from build123d import *

# Parameters (mm, degrees)
F0_W     = 38.1
F0_H     = 3.175
F1_DEPTH = 15.875
F2_W     = 38.1
F2_H     = 3.175
F3_DEPTH = 2.54
F5_DEPTH = 25.4
F6_R     = 3.2385
F7_DEPTH = 101.6


with BuildPart() as f1:
    # F0 (on Top) → F1 (new body)
    with BuildSketch(Plane.XY):
        with BuildLine():
            Line((-43.00682, 50.395912), (-46.18182, 50.395912))
            Line((-46.18182, 50.395912), (-46.18182, -35.329088))
            ThreePointArc((-46.18182, -35.329088), (-44.321948, -39.819216), (-39.83182, -41.679088))
            Line((-39.83182, -41.679088), (-39.83182, -38.504088))
            ThreePointArc((-39.83182, -38.504088), (-42.076884, -37.574152), (-43.00682, -35.329088))
            Line((-43.00682, -35.329088), (-43.00682, 50.395912))
        make_face()
        with Locations((-20.78182, -40.091588)):
            Rectangle(F0_W, F0_H)
        with BuildLine():
            Line((-1.73182, -38.504088), (-1.73182, -41.679088))
            ThreePointArc((-1.73182, -41.679088), (2.758308, -39.819216), (4.61818, -35.329088))
            Line((4.61818, -35.329088), (4.61818, 50.395912))
            Line((4.61818, 50.395912), (1.44318, 50.395912))
            Line((1.44318, 50.395912), (1.44318, -35.329088))
            ThreePointArc((1.44318, -35.329088), (0.513244, -37.574152), (-1.73182, -38.504088))
        make_face()
    extrude(amount=F1_DEPTH)

    # F2 (on face) → F3 (join)
    with BuildSketch(Plane.XY.offset(15.875)):
        with Locations((-20.78182, -40.091588)):
            Rectangle(F2_W, F2_H)
    extrude(amount=F3_DEPTH)

    # F4 (on face) → F5 (cut)
    with BuildSketch(Plane.XZ.offset(41.679088)):
        Polygon((-39.83182, 18.415), (-39.83182, 15.875), (-37.29182, 18.415), align=None)
        Polygon((-1.73182, 18.415), (-4.207504, 18.415), (-1.73182, 15.875), align=None)
    extrude(amount=-F5_DEPTH, mode=Mode.SUBTRACT)

    # F6 (on face) → F7 (cut)
    with BuildSketch(Plane(origin=(-46.18182, 0, 0), x_dir=(0, -1, 0), z_dir=(-1, 0, 0))):
        with Locations((-42.471112, 7.9502)):
            Circle(F6_R)
    extrude(amount=-F7_DEPTH, mode=Mode.SUBTRACT)


solid = f1.part
Read the model definition and answer for the solid it produces. Units are mm, in the model's axes. A direction names the side the tool comes from. Give positions to 0.01 mm unless a question says otherwise; leave off trailing zeros. Loops run counter-clockwise (first coordinate to the right, second up) from the corner with the lowest first, then second, coordinate; pieces in that order, holes last. Notation, with made-up numbers: (61, 59) -> (72, 59) arc R16 ccw to (72, 75) -> close; hole circle Ø6 at (41.5, 70.5). An arc over 180 degrees is marked (long way). Answer as CSV lines item,"result".
Item 1: For faces 1 (the face through (3, 50.396, 8)), 2 (the face through (-43.007, 7, 8)), determine the directions among +Z, -Z, +X, -X, +Y, -Y from which every point of the face is accessible in a straight line to the end or side of a thin tool.
Returned:
face 1,"+Z, -Z, +X, -X, +Y"
face 2,"+Z, -Z, +Y"
Item 2: Find section A-A on y = -23.5. Give the vertices of the cut face in (x, z) (3 decimals), plus the area to 3 significant figures.
Returned:
outline,"(-46.182, 0) -> (-43.007, 0) -> (-43.007, 15.875) -> (-46.182, 15.875) -> close; (1.443, 0) -> (4.618, 0) -> (4.618, 15.875) -> (1.443, 15.875) -> close"
area,"101 mm²"
Item 3: Find section D-D on z = 2. Give the vertices of the cut face in (x, y) (3 decimals), plus the area to 3 significant figures.
Returned:
outline,"(-46.182, -35.329) arc R6.35 ccw to (-39.832, -41.679) -> (-1.732, -41.679) arc R6.35 ccw to (4.618, -35.329) -> (4.618, 50.396) -> (1.443, 50.396) -> (1.443, -35.329) arc R3.175 cw to (-1.732, -38.504) -> (-39.832, -38.504) arc R3.175 cw to (-43.007, -35.329) -> (-43.007, 50.396) -> (-46.182, 50.396) -> close"
area,"713 mm²"
Item 4: Determine the mould class of faces 3 (the face through (-2.987, -40.114, 17.163)), 4 (the face through (-21, -41.679, 9)), 5 (the face through (0.538, -37.549, 7.826)) for opening direction X: +X half, -X half, draft (parallel to the pull), parting line (faces both ways), or undercut.
Returned:
face 3,"+X half"
face 4,"draft"
face 5,"undercut"
Item 5: Consider line 1 (X direction, y = 42.5, z = 13); line 2 (Y direction, x = -6, z = 9.5); line 3 (Z direction, x = 2, y = -5.5) (3 decimals). Determine where each line is inside the solid, lowest interval first. Write a range as [from, to].
Returned:
line 1,"x = [-46.18, -43.01], [1.44, 4.62]"
line 2,"y = [-41.68, -38.5]"
line 3,"z = [0, 15.875]"
Item 6: Find section B-B on z = 10.25. Give the vertices of the cut face in (x, y) (3 decimals).
Returned:
outline,"(-46.182, -35.329) arc R6.35 ccw to (-39.832, -41.679) -> (-1.732, -41.679) arc R6.35 ccw to (4.618, -35.329) -> (4.618, 40.191) -> (1.443, 40.191) -> (1.443, -35.329) arc R3.175 cw to (-1.732, -38.504) -> (-39.832, -38.504) arc R3.175 cw to (-43.007, -35.329) -> (-43.007, 40.191) -> (-46.182, 40.191) -> close; (-46.182, 44.751) -> (-43.007, 44.751) -> (-43.007, 50.396) -> (-46.182, 50.396) -> close; (1.443, 44.751) -> (4.618, 44.751) -> (4.618, 50.396) -> (1.443, 50.396) -> close"
Item 7: Each of these flat-tipped pins is pushed along its axis until it touches: pin 1 (5 mm diameter, centred on x = 2.5, y = -1, fed in from +Z) (3 decimals); pin 2 (5.5 mm diameter, centred on x = -18.5, z = 7, fed in from +Y); pin 3 (8.5 mm diameter, centred on y = 42.47, z = 7.95, fed in from +X). Where does it stop, or does it pass through?
Returned:
pin 1,"stops at z = 15.875"
pin 2,"stops at y = -38.5"
pin 3,"stops at x = 4.62"
Item 8: Find section C-C on y = 40.5. Give the vertices of the cut face in (x, z) (3 decimals).
Returned:
outline,"(-46.182, 0) -> (-43.007, 0) -> (-43.007, 5.381) -> (-46.182, 5.381) -> close; (-46.182, 10.52) -> (-43.007, 10.52) -> (-43.007, 15.875) -> (-46.182, 15.875) -> close; (1.443, 0) -> (4.618, 0) -> (4.618, 5.381) -> (1.443, 5.381) -> close; (1.443, 10.52) -> (4.618, 10.52) -> (4.618, 15.875) -> (1.443, 15.875) -> close"
